```python
from build123d import *

# Parameters (mm, degrees)
F0_W      = 67.1
F0_H      = 138.3
F1_DEPTH  = 3.55
F2_R      = 5
F3_T      = -2.5
F4_W      = 20.0819657184
F4_H      = 7.4590183794
F5_DEPTH  = 12.5
F7_R      = 10.7534144168
F8_DEPTH  = 12.5
F6_W      = 22.7594478056
F6_H      = 3.1675179489
F9_DEPTH  = 12.5
F10_W     = 3.7042096956
F10_H     = 9.4521231949
F11_DEPTH = 12.5


with BuildPart() as f1:
    # F0 (on Front) → F1 (new body, symmetric)
    with BuildSketch(Plane.XZ):
        with Locations((0, -3.435843619)):
            Rectangle(F0_W, F0_H)
    extrude(amount=F1_DEPTH, both=True)

    # F2
    f2_edges = [f1.edges().sort_by_distance(p)[0] for p in [
        (33.55, 0, 65.714156),
        (33.55, 0, -72.585844),
        (-33.55, 0, -72.585844),
        (-33.55, 0, 65.714156),
    ]]
    fillet(f2_edges, radius=F2_R)

    # F3
    f3_openings = [f1.faces().sort_by_distance(p)[0] for p in [
        (0, -3.55, -3.435844),
    ]]
    offset(amount=F3_T, openings=f3_openings)

    # F4 (on face) → F5 (cut, symmetric)
    with BuildSketch(Plane.XZ.offset(-1.05)):
        with Locations((17.2131143045, 54.9385268241)):
            Rectangle(F4_W, F4_H)
    extrude(amount=F5_DEPTH, both=True, mode=Mode.SUBTRACT)

    # F7 (on face) → F8 (cut, symmetric)
    with BuildSketch(Plane.XZ.offset(-1.05)):
        with Locations((0, 14.4877051935)):
            Circle(F7_R)
    extrude(amount=F8_DEPTH, both=True, mode=Mode.SUBTRACT)

    # F6 (on face) → F9 (cut, symmetric)
    with BuildSketch(Plane(origin=(0, 0, -72.585843619), x_dir=(1, 0, 0), z_dir=(0, 0, -1))):
        with Locations((0.5839481018, 0.0267331488)):
            Rectangle(F6_W, F6_H)
    extrude(amount=F9_DEPTH, both=True, mode=Mode.SUBTRACT)

    # F10 (on face) → F11 (cut, symmetric)
    with BuildSketch(Plane(origin=(-33.55, 0, 0), x_dir=(0, -1, 0), z_dir=(-1, 0, 0))):
        with Locations((-0.4275311367, 46.8149799854)):
            Rectangle(F10_W, F10_H)
    extrude(amount=F11_DEPTH, both=True, mode=Mode.SUBTRACT)


solid = f1.part
```
Here's how the part is built. I have some questions about the finished solid (model axes, mm). A direction names the side the tool comes from. Give positions to 0.01 mm unless a question says otherwise; leave off trailing zeros. Loops run counter-clockwise (first coordinate to the right, second up) from the corner with the lowest first, then second, coordinate; pieces in that order, holes last. Notation, with made-up numbers: M 32.25,-23 L 74.25,-23 A17 cw 74.25,-7 Z; hole C 70,-35 d2. An arc over 180 degrees is marked long. Put each result on its own line as item: value. Start each with the question number.
(1) I want a section at A-A on x = 0. Please give me the cut outline in (y, z), then the cut area to 3 significant figures.
(2) I need wall thicknesses on line 1 along Z through (x, y) = (0, 2.45); line 2 along X through (y, z) = (0, -63.5); line 3 along Z through (x, y) = (-13, -0.75). Which ranges of each line are inside material? Lowest first, please. Write a range as [from, to].
(3) I want a section at B-B on x = 13.5. Please give me the cut outline in (y, z).
(4) I want a section at C-C on z = 37. Please give me the cut outline in (x, y).
(5) I want a section at D-D on x = -7.5. Please give me the cut outline in (y, z), then the cut area to 3 significant figures.
(6) If we mould it in two halves opening along Z, with no side actions, what happens to faces 5 (the flat face through (31.05, -1, -4)), 6 (the cylindrical face through (-32.124, -0.05, -71.082)), 7 (the flat face through (0, 3.55, -2)), 8 (the cylindrical face through (30.34, -1.28, -69.33))? For each: +Z half, -Z half, draft (parallel to the pull), parting line (faces both ways), or undercut.
(7) For faces 1 (the flat face through (17, 2, 51.209)), 2 (the cylindrical face through (-30.3, -1.2, 62.5)), 3 (the flat face through (-27, 2.28, 47)), 4 (the flat face through (0, -2, -72.586)), which set-ups out of +Z, -Z, +X, -X, +Y, -Y let a thin tool reach every point of the face, with its end or its side?
(8) Will these pins go through, and if not, where does the flat tip stop? pin 1 Ø1 at (x, z) = (11.5, 29) entering from -Y; pin 2 Ø7.5 at (x, z) = (-25.5, 47) entering from -Y; pin 3 Ø1 at (y, z) = (1.5, 45.5) entering from -X.
Answer block:
1. outline: M -3.55,-72.59 L -1.61,-72.59 L -1.61,-70.09 L -3.55,-70.09 Z; M -3.55,63.21 L 1.05,63.21 L 1.05,25.24 L 3.55,25.24 L 3.55,65.71 L -3.55,65.71 Z; M 1.05,-60.09 L 1.56,-60.09 L 1.56,-72.59 L 3.55,-72.59 L 3.55,3.73 L 1.05,3.73 Z
1. area: 302 mm^2
2. line 1: [-72.59, 3.73], [25.24, 65.71]
2. line 2: [-33.55, -31.05], [31.05, 33.55]
2. line 3: [-72.59, -70.09], [63.21, 65.71]
3. outline: M -3.55,-72.59 L 3.55,-72.59 L 3.55,51.21 L 1.05,51.21 L 1.05,-70.09 L -3.55,-70.09 Z; M -3.55,63.21 L 1.05,63.21 L 1.05,58.67 L 3.55,58.67 L 3.55,65.71 L -3.55,65.71 Z
4. outline: M -33.55,-3.55 L -31.05,-3.55 L -31.05,1.05 L 31.05,1.05 L 31.05,-3.55 L 33.55,-3.55 L 33.55,3.55 L -33.55,3.55 Z
5. outline: M -3.55,-72.59 L -1.61,-72.59 L -1.61,-70.09 L -3.55,-70.09 Z; M -3.55,63.21 L 1.05,63.21 L 1.05,22.19 L 3.55,22.19 L 3.55,65.71 L -3.55,65.71 Z; M 1.05,-60.09 L 1.56,-60.09 L 1.56,-72.59 L 3.55,-72.59 L 3.55,6.78 L 1.05,6.78 Z
5. area: 317 mm^2
6. face 5: undercut
6. face 6: -Z half
6. face 7: draft
6. face 8: undercut
7. face 1: +Y, -Y
7. face 2: -Y
7. face 3: -X
7. face 4: -Z, +X, -X, +Y, -Y
8. pin 1: y = 1.05
8. pin 2: y = 2.28
8. pin 3: x = -21.05
